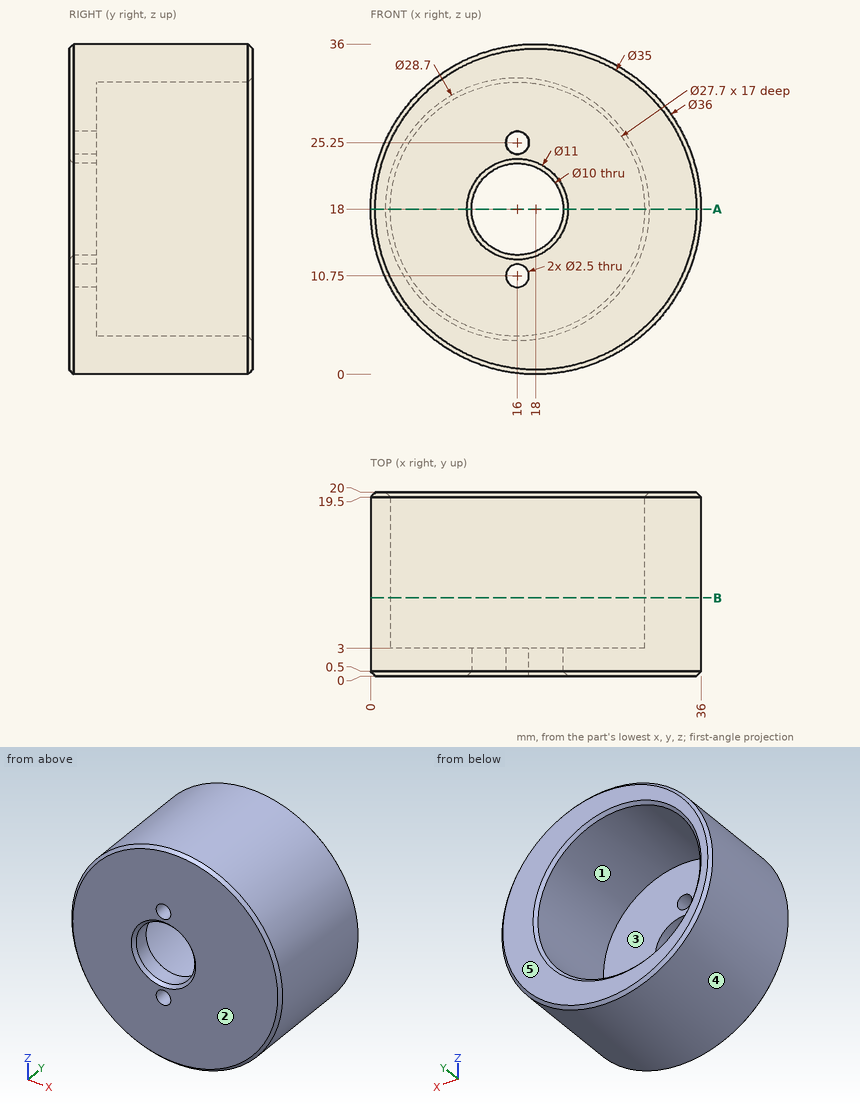
Part print with two shaded views. Sizes in mm from the minimum x, y, z corner. A direction names the side the tool comes from. Give positions to 0.01 mm unless a question says otherwise; leave off trailing zeros. Order: outer loops, then holes, each group sorted by start corner. A loop starts at its lowest first (then second) coordinate and runs counter-clockwise, first axis right, second up.
(1) Mould opens along Z. For the marked faces 3, 4 and 5 say: released by +Z, released by -Z, zero draft, split by the parting line, or undercut.
(2) Tool access for the marked faces 1 and 2: list every direction of +Z, -Z, +X, -X, +Y, -Y with a clear straight run to the whole face (end or side of a thin tool).
(3) Saw through at A-A, the plane z = 18. Give the cut face in (x, y), then the cut area to 3 significant figures.
(4) Drill centre lines: L1, parallel to X at y = 2.1, z = 18; L2, parallel to Z at x = 16, y = 1.65; L3, parallel to Z at x = 11, y = 6.25. Where is each one in solid material? Low to high.
(5) Saw through at B-B, the plane y = 8.5. Give the cut face in (x, z).
(6) Flat gauge pins, fed straight in: pin 1 (1.5 mm diameter, centred on y = 13.5, z = 9, fed in from -X); pin 2 (3 mm diameter, centred on x = 22.5, y = 10, fed in from +Z); pin 3 (3 mm diameter, centred on x = 16, z = 10.75, fed in from -Y); pin 4 (3 mm diameter, centred on y = 4.5, z = 9.5, fed in from -X). Where does each tip first touch, or does it go through?
Results found:
1. face 3: undercut
1. face 4: split by the parting line
1. face 5: zero draft
2. face 1: +Y
2. face 2: +Z, -Z, +X, -X, -Y
3. outline: (0, 0.5) - (0.5, 0) - (10.5, 0) - (11, 0.5) - (11, 3) - (2.15, 3) - (2.15, 19.5) - (1.65, 20) - (0.5, 20) - (0, 19.5) - close; (21, 0.5) - (21.5, 0) - (35.5, 0) - (36, 0.5) - (36, 19.5) - (35.5, 20) - (30.35, 20) - (29.85, 19.5) - (29.85, 3) - (21, 3) - close
3. area: 218 mm2
4. L1: x = 0 to 11, 21 to 36
4. L2: z = 0.11 to 9.5, 12 to 13, 23 to 24, 26.5 to 35.89
4. L3: z = 1.42 to 5.08, 30.92 to 34.58
5. outline: circle Ø36 at (18, 18); hole circle Ø27.7 at (16, 18)
6. pin 1: stops at x = 2
6. pin 2: stops at z = 35.75
6. pin 3: stops at y = 0
6. pin 4: stops at x = 1.42
